Autodesk Inventor part; units mm, degrees
ref_plane "YZ Plane" through (0, 0, 0) normal (1, 0, 0) x (0, 1, 0)
ref_plane "XZ Plane" through (0, 0, 0) normal (0, 1, 0) x (-1, 0, 0)
ref_plane "XY Plane" through (0, 0, 0) normal (0, 0, 1) x (1, 0, 0)
sketch "Esquisse1" plane through (0, 0, 0) normal (0, 1, 0) x (-1, 0, 0)
  line L0 (50, 50) -> (-50, 50)
  line L1 (-50, 50) -> (-50, -50)
  line L2 (-50, -50) -> (50, -50)
  line L3 (50, -50) -> (50, 50)
  point P0 (0, 0)
  dimension "d0" = 100
  dimension "d1" = 100
  dimension "d17" = 50
  dimension "d18" = 50
extrude "Extrusion1" add sketch "Esquisse1" along normal blind 2
sketch "Esquisse2" plane through (0, 2, 0) normal (0, 1, 0) x (1, 0, 0)
  line L0 (50, -50) -> (50, 50)
  line L1 (-50, -50) -> (50, -50)
  arc A0 (36.32, -38.1309) -> (27.6597, -38.1165) centre (32, -32) ccw
  line L2 (27.68, -29.4825) -> (32.0203, -27)
  line L3 (32.0203, -27) -> (36.3403, -29.5175)
  line L4 (36.3403, -29.5175) -> (36.32, -34.5175)
  line L5 (27.6597, -34.4825) -> (27.68, -29.4825)
  line L6 (27.6597, -34.4825) -> (27.6597, -38.1165)
  line L7 (36.32, -34.5175) -> (36.32, -38.1309)
  line L8 (53.6963, 0) -> (-74.6388, 0)
  line L9 (0, -61.7794) -> (0, 59.6738)
  arc A1 (-27.6597, -38.1165) -> (-36.32, -38.1309) centre (-32, -32) ccw
  line L10 (-27.68, -29.4825) -> (-32.0203, -27)
  line L11 (-32.0203, -27) -> (-36.3403, -29.5175)
  line L12 (-36.3403, -29.5175) -> (-36.32, -34.5175)
  line L13 (-27.6597, -34.4825) -> (-27.68, -29.4825)
  line L14 (-27.6597, -34.4825) -> (-27.6597, -38.1165)
  line L15 (-36.32, -34.5175) -> (-36.32, -38.1309)
  arc A2 (27.6597, 38.1165) -> (36.32, 38.1309) centre (32, 32) ccw
  line L16 (27.68, 29.4825) -> (32.0203, 27)
  line L17 (32.0203, 27) -> (36.3403, 29.5175)
  line L18 (36.3403, 29.5175) -> (36.32, 34.5175)
  line L19 (27.6597, 34.4825) -> (27.68, 29.4825)
  line L20 (27.6597, 34.4825) -> (27.6597, 38.1165)
  line L21 (36.32, 34.5175) -> (36.32, 38.1309)
  arc A3 (-36.32, 38.1309) -> (-27.6597, 38.1165) centre (-32, 32) ccw
  line L22 (-27.68, 29.4825) -> (-32.0203, 27)
  line L23 (-32.0203, 27) -> (-36.3403, 29.5175)
  line L24 (-36.3403, 29.5175) -> (-36.32, 34.5175)
  line L25 (-27.6597, 34.4825) -> (-27.68, 29.4825)
  line L26 (-27.6597, 34.4825) -> (-27.6597, 38.1165)
  line L27 (-36.32, 34.5175) -> (-36.32, 38.1309)
  point P0 (0, 0)
  dimension "d6" = 18
  dimension "d7" = 18
  dimension "d8" = 15
  dimension "d9" = 5
extrude "Extrusion2" add sketch "Esquisse2" along normal blind 4 contours L7 L4 L3 L2 L5 L6 A0 | L14 L13 L10 L11 L12 L15 A1 | L20 L19 L16 L17 L18 L21 A2 | L27 L24 L23 L22 L25 L26 A3
sketch "Esquisse4" plane through (0, 6, 0) normal (0, 1, 0) x (1, 0, 0)
  arc A0 (36.32, -38.1309) -> (27.6597, -38.1165) centre (32, -32) ccw
  line L0 (27.6597, -38.1165) -> (36.3403, -38.1165)
  line L1 (53.7761, 0) -> (-84.9694, 0)
  line L2 (0, -51.9111) -> (0, 71.3221)
  arc A1 (-27.6597, -38.1165) -> (-36.32, -38.1309) centre (-32, -32) ccw
  line L3 (-27.6597, -38.1165) -> (-36.3403, -38.1165)
  arc A2 (27.6597, 38.1165) -> (36.32, 38.1309) centre (32, 32) ccw
  line L4 (27.6597, 38.1165) -> (36.3403, 38.1165)
  arc A3 (-36.32, 38.1309) -> (-27.6597, 38.1165) centre (-32, 32) ccw
  line L5 (-27.6597, 38.1165) -> (-36.3403, 38.1165)
  point P0 (0, 0)
extrude "Extrusion3" add sketch "Esquisse4" along normal blind 3
sketch "Esquisse5" plane through (0, 9, 0) normal (0, 1, 0) x (1, 0, 0)
  circle A0 centre (32, -32) radius 2
  arc A1 (36.3403, -38.1165) -> (27.6597, -38.1165) centre (32, -32) ccw
  line L0 (0, -51.4977) -> (0, 66.0278)
  line L1 (54.9768, 0) -> (-89.9714, 0)
  circle A2 centre (-32, -32) radius 2
  arc A3 (-27.6597, -38.1165) -> (-36.3403, -38.1165) centre (-32, -32) ccw
  circle A4 centre (32, 32) radius 2
  arc A5 (27.6597, 38.1165) -> (36.3403, 38.1165) centre (32, 32) ccw
  circle A6 centre (-32, 32) radius 2
  arc A7 (-36.3403, 38.1165) -> (-27.6597, 38.1165) centre (-32, 32) ccw
  point P0 (0, 0)
  dimension "d14" = 4
extrude "Extrusion4" cut sketch "Esquisse5" against normal through all
ref_plane "Plan de construction3" through (0, 0, 50) normal (1, 0, 0) x (0, 0, -1)
ref_plane "Plan de construction4" through (-50, 0, 0) normal (0, 0, 1) x (1, 0, 0)
sketch "Esquisse6" plane through (0, 0, 0) normal (0, -1, 0) x (1, 0, 0)
  circle A0 centre (20.8597, 20.8597) radius 1.6
  circle A1 centre (20.8597, -20.8597) radius 1.6
  circle A2 centre (-20.8597, 20.8597) radius 1.6
  circle A3 centre (-20.8597, -20.8597) radius 1.6
  point P0 (0, 0)
extrude "Extrusion5" cut sketch "Esquisse6" against normal through all
properties part number "support-balise"
Geometry: final body of the model. Coordinates: model frame, mm. A direction names the side the tool comes from. Coordinates: 2 decimals unless noted, no trailing zeros. Write each loop counter-clockwise with the first axis right and the second up, starting at its lowest first coordinate (ties: lowest second). Pieces come first, ordered by that corner, then holes. Notation, with made-up numbers: M 39.25,-7.5 L 72.25,-7.5 A29 cw 72.25,20.5 Z; hole C 46.25,45.25 d8. An arc over 180 degrees is marked long. Use CSV: the item, a comma, the result in double quotes. Start each with the question number.
1. First-contact query: P1, Ø3.5, axis at x = 32, z = -32, coming from the +Y side; P2, Ø3, axis at x = 34.5, y = 6, coming from the -Z side; P3, Ø1.8, axis at y = 3, z = -37, coming from the -X side; P4, Ø1.5, axis at x = -26, y = 6.5, coming from the -Z side. Flat tips, straight axial feed; report the tip coordinate or a pass-through.
2. Reachability of faces 1 (the face through (32, 6, 35)), 2 (the face through (27.66, 4, -36)), 3 (the face through (31.747, 5.451, 24.504)) from +Z, -Z, +X, -X, +Y, -Y: full face, straight path, thin tool, end or side. Return the list, or none.
3. Cut plane B-B on z = -43. Return the cut outline in (x, y), plus the area to 3 significant figures.
4. Cut plane C-C on z = 32. Count the separate pieces of the cut face and the enclosed holes in it, plus the area to 3 significant figures.
5. Ray query, probe 1 along Z at (x, y) = (-32, 1.5); probe 2 along Z at (x, y) = (32, 6.8). Return the intervals inside material, ascending.
6. Mould query, pull axis Z, two halves, no side actions, for faces 4 (the face through (-36.32, 4, -36)), 5 (the face through (32, 7, -38.116)), 6 (the face through (-31.077, 7.521, -30.226)). Classes: pulls with the +Z half, pulls with the -Z half, needs draft (parallel to the pull), parting line crosses it, or undercut.
7. Cut plane A-A on y = 4. Return the cut outline in (x, z).
Entries:
1,P1,"through"
1,P2,"z = -38.12"
1,P3,"x = -38.28"
1,P4,"z = -37.36"
2,face 1,"+Z"
2,face 2,"-Z"
2,face 3,"+Y"
3,outline,"M -50,0 L 50,0 L 50,2 L -50,2 Z"
3,area,"200 mm²"
4,separate pieces,"3"
4,enclosed holes,"0"
4,area,"301 mm²"
5,probe 1,"-50 to -34, -30 to 30, 34 to 50"
5,probe 2,"-38.12 to -34, -30 to -24.5, 24.5 to 30, 34 to 38.12"
6,face 4,"needs draft"
6,face 5,"pulls with the -Z half"
6,face 6,"undercut"
7,outline,"M -36.34,-29.52 L -32.02,-27 L -27.68,-29.48 L -27.66,-34.48 L -27.66,-38.12 A7.5 ccw long -36.32,-38.13 L -36.32,-34.52 Z; M -36.34,29.52 L -36.32,34.52 L -36.32,38.13 A7.5 ccw long -27.66,38.12 L -27.66,34.48 L -27.68,29.48 L -32.02,27 Z; M 27.66,-38.12 L 27.66,-34.48 L 27.68,-29.48 L 32.02,-27 L 36.34,-29.52 L 36.32,-34.52 L 36.32,-38.13 A7.5 ccw long Z; M 27.66,34.48 L 27.66,38.12 A7.5 ccw long 36.32,38.13 L 36.32,34.52 L 36.34,29.52 L 32.02,27 L 27.68,29.48 Z"
